Geometry check sheet. Reference: the model listing, model coordinates, mm. A direction names the side the tool comes from. Coordinates: 2 decimals unless noted, no trailing zeros. Loops run counter-clockwise (first coordinate to the right, second up) from the corner with the lowest first, then second, coordinate; pieces in that order, holes last.
from build123d import *

# Parameters (mm, degrees)
EXTRUDE_1_DEPTH = 26.4


with BuildPart() as part:
    # Эскиз1 → Бобышка-Вытянуть1 (new body)
    with BuildSketch(Plane(origin=(0, 0, 0), x_dir=(1, 0, 0), z_dir=(0, 1, 0))):
        with BuildLine():
            Line((0, -7.366273292), (0, -1.430737225))
            Line((0, -1.430737225), (-23.119998808, -1.430737225))
            Line((-23.119998808, -1.430737225), (-23.119998808, -7.366273292))
            ThreePointArc((-23.119998808, -7.366273292), (-23.204411997, -7.465051079), (-23.315139834, -7.397065907))
            Line((-23.315139834, -7.397065907), (-25.151536602, -1.723086212))
            ThreePointArc((-25.151536602, -1.723086212), (-25.246516215, -1.653878958), (-25.341718752, -1.722779233))
            Line((-25.341718752, -1.722779233), (-27.163713043, -7.290838427))
            ThreePointArc((-27.163713043, -7.290838427), (-27.276953731, -7.358068766), (-27.358630238, -7.254761845))
            Line((-27.358630238, -7.254761845), (-27.147073457, -3.009330281))
            ThreePointArc((-27.147073457, -3.009330281), (-27.186129834, -2.924974677), (-27.277742143, -2.909212268))
            Line((-27.277742143, -2.909212268), (-28.656433819, -3.355429045))
            Line((-28.656433819, -3.355429045), (-33.693480219, -7.637416988))
            ThreePointArc((-33.693480219, -7.637416988), (-33.821863766, -7.638385786), (-33.84539196, -7.51217288))
            Line((-33.84539196, -7.51217288), (-32.027666378, -4.283069467))
            Line((-32.027666378, -4.283069467), (-33.457933536, -4.683052776))
            ThreePointArc((-33.457933536, -4.683052776), (-33.57629105, -4.627262362), (-33.538118808, -4.502106653))
            Line((-33.538118808, -4.502106653), (-28.656434415, -1.430737225))
            ThreePointArc((-28.656434415, -1.430737225), (-27.22569719, 0), (-28.656434415, 1.430737225))
            Line((-28.656434415, 1.430737225), (-33.538118808, 4.502106653))
            ThreePointArc((-33.538118808, 4.502106653), (-33.57629105, 4.627262362), (-33.457933536, 4.683052776))
            Line((-33.457933536, 4.683052776), (-32.027666378, 4.283069467))
            Line((-32.027666378, 4.283069467), (-33.84539196, 7.51217288))
            ThreePointArc((-33.84539196, 7.51217288), (-33.821862569, 7.638384319), (-33.693480241, 7.637416132))
            Line((-33.693480241, 7.637416132), (-28.656433494, 3.355428597))
            Line((-28.656433494, 3.355428597), (-27.277741782, 2.909211931))
            ThreePointArc((-27.277741782, 2.909211931), (-27.186129475, 2.924974348), (-27.147073104, 3.009329955))
            Line((-27.147073104, 3.009329955), (-27.358630229, 7.254761502))
            ThreePointArc((-27.358630229, 7.254761502), (-27.27695373, 7.35806843), (-27.163713037, 7.2908381))
            Line((-27.163713037, 7.2908381), (-25.341718295, 1.722779053))
            ThreePointArc((-25.341718295, 1.722779053), (-25.246515752, 1.653878786), (-25.151536145, 1.723086048))
            Line((-25.151536145, 1.723086048), (-23.315139837, 7.397065891))
            ThreePointArc((-23.315139837, 7.397065891), (-23.204412005, 7.465051072), (-23.119998808, 7.366273292))
            Line((-23.119998808, 7.366273292), (-23.119998808, 1.430737225))
            Line((-23.119998808, 1.430737225), (0, 1.430737225))
            Line((0, 1.430737225), (0, 7.366273292))
            ThreePointArc((0, 7.366273292), (0.084413196, 7.465051072), (0.195141029, 7.397065891))
            Line((0.195141029, 7.397065891), (2.031537337, 1.723086048))
            ThreePointArc((2.031537337, 1.723086048), (2.126516944, 1.653878786), (2.221719487, 1.722779053))
            Line((2.221719487, 1.722779053), (4.043714229, 7.2908381))
            ThreePointArc((4.043714229, 7.2908381), (4.156954922, 7.35806843), (4.238631421, 7.254761502))
            Line((4.238631421, 7.254761502), (4.027074296, 3.009329955))
            ThreePointArc((4.027074296, 3.009329955), (4.066130667, 2.924974348), (4.157742974, 2.909211931))
            Line((4.157742974, 2.909211931), (5.536434686, 3.355428597))
            Line((5.536434686, 3.355428597), (10.573481433, 7.637416132))
            ThreePointArc((10.573481433, 7.637416132), (10.701863761, 7.638384319), (10.725393152, 7.51217288))
            Line((10.725393152, 7.51217288), (8.90766757, 4.283069467))
            Line((8.90766757, 4.283069467), (10.337934728, 4.683052776))
            ThreePointArc((10.337934728, 4.683052776), (10.456292242, 4.627262362), (10.41812, 4.502106653))
            Line((10.41812, 4.502106653), (5.536435606, 1.430737225))
            ThreePointArc((5.536435606, 1.430737225), (4.105698382, 0), (5.536435606, -1.430737225))
            Line((5.536435606, -1.430737225), (10.41812, -4.502106653))
            ThreePointArc((10.41812, -4.502106653), (10.456292242, -4.627262362), (10.337934728, -4.683052776))
            Line((10.337934728, -4.683052776), (8.90766757, -4.283069467))
            Line((8.90766757, -4.283069467), (10.725393152, -7.51217288))
            ThreePointArc((10.725393152, -7.51217288), (10.701864958, -7.638385786), (10.573481411, -7.637416988))
            Line((10.573481411, -7.637416988), (5.536435011, -3.355429045))
            Line((5.536435011, -3.355429045), (4.157743335, -2.909212268))
            ThreePointArc((4.157743335, -2.909212268), (4.066131026, -2.924974677), (4.027074648, -3.009330281))
            Line((4.027074648, -3.009330281), (4.23863143, -7.254761845))
            ThreePointArc((4.23863143, -7.254761845), (4.156954922, -7.358068766), (4.043714235, -7.290838427))
            Line((4.043714235, -7.290838427), (2.221719944, -1.722779233))
            ThreePointArc((2.221719944, -1.722779233), (2.126517406, -1.653878958), (2.031537794, -1.723086212))
            Line((2.031537794, -1.723086212), (0.195141026, -7.397065907))
            ThreePointArc((0.195141026, -7.397065907), (0.084413188, -7.465051079), (0, -7.366273292))
        make_face()
    extrude(amount=EXTRUDE_1_DEPTH)


solid = part.part
1) Access from +Z, -Z, +X, -X, +Y, -Y to the whole of each face (thin tool, end or side, straight path). Record for faces 4 (the flat face through (4.13, 13.02, 5.1)), 5 (the flat face through (8.09, 13.015, 5.526)), 6 (the flat face through (7.943, 13.015, 2.945)), 7 (the flat face through (0, 13, -4)).
Data:
face 4: +Y, -Y
face 5: +Z, +Y, -Y
face 6: +X, +Y, -Y
face 7: -Z, +Y, -Y
2) Section check C-C on x = -8.5. Record the cut outline in (y, z).
Data:
outline: (0, -1.43) - (26.4, -1.43) - (26.4, 1.43) - (0, 1.43) - close
3) Mould release check, pull along X, two halves, no side actions. Record for faces 1 (the cylindrical face through (-27.226, 13.015, 0.031)), 2 (the cylindrical face through (4.106, 13.015, -0.031)), 3 (the flat face through (-26.24, 13.02, 4.47)): +X half, -X half, draft (parallel to the pull), parting line (faces both ways), or undercut.
Data:
face 1: -X half
face 2: +X half
face 3: undercut
4) Material ranges on probe 1 along X at (y, z) = (17.5, -2.75); probe 2 along X at (y, z) = (4, -3.75); probe 3 along X at (y, z) = (12.25, 6), recorded low to high.
Data:
probe 1: x = -30.75 to -25.68, -24.82 to -23.12, 0 to 1.7, 2.56 to 7.63
probe 2: x = -32.34 to -29.12, -27.18 to -26.01, -24.5 to -23.12, 0 to 1.38, 2.89 to 4.06, 6 to 9.22
probe 3: x = -32.99 to -31.77, -27.3 to -26.74, -23.77 to -23.12, 0 to 0.65, 3.62 to 4.18, 8.65 to 9.87
5) Section check B-B on z = 0. Record the cut outline in (x, y), and give its area (3 significant figures).
Data:
outline: (-27.23, 0) - (4.11, 0) - (4.11, 26.4) - (-27.23, 26.4) - close
area: 827 mm2
6) Depth check by flat-ended pin: pin 1 (4.5 mm diameter, centred on y = 19, z = -3, fed in from -X); pin 2 (1.8 mm diameter, centred on y = 11.5, z = 3.5, fed in from +X); pin 3 (1 mm diameter, centred on y = 3, z = -1.5, fed in from -X). Enter the tip coordinate at first touch or a pass-through.
Data:
pin 1: stops at x = -33.58
pin 2: stops at x = 10.26
pin 3: stops at x = -29.56
7) Section check A-A on z = 5.5. Record the cut outline in (x, y).
Data:
outline: (-32.71, 0) - (-31.18, 0) - (-31.18, 26.4) - (-32.71, 26.4) - close; (-27.27, 0) - (-26.58, 0) - (-26.58, 26.4) - (-27.27, 26.4) - close; (-23.93, 0) - (-23.12, 0) - (-23.12, 26.4) - (-23.93, 26.4) - close; (0, 0) - (0.81, 0) - (0.81, 26.4) - (0, 26.4) - close; (3.46, 0) - (4.15, 0) - (4.15, 26.4) - (3.46, 26.4) - close; (8.06, 0) - (9.59, 0) - (9.59, 26.4) - (8.06, 26.4) - close
